Input: part model. Units: mm. Frame: model coordinates. A direction names the side the tool comes from. Give positions to 0.01 mm unless a question says otherwise; leave off trailing zeros. Loops run counter-clockwise (first coordinate to the right, second up) from the corner with the lowest first, then second, coordinate; pieces in that order, holes last. Notation, with made-up numbers: M 1,29 L 15,29 A17 ccw 15,39 Z; hole C -36.5,-12 d11. An arc over 180 degrees is marked long. Use CSV: the item, a comma, the result in double quotes. Start each with the question number.
Q1. Reachability of faces 4 (the flat face through (9.525, 0, 266)), 5 (the flat face through (-10, -2, 539.75)) from +Z, -Z, +X, -X, +Y, -Y: full face, straight path, thin tool, end or side. Return the list, or none.
Q2. Material intervals for line 1 along X through (y, z) = (6, 145) (3 decimals); line 2 along X through (y, z) = (-23, 533); line 3 along Y through (x, z) = (2, 227) (3 decimals), sorted ascending.
Q3. Pin query (flat end, axial travel): pin 1 (2 mm diameter, centred on y = 0, z = 148.968, fed in from -X) (3 decimals). Return the tip coordinate at first contact, or that it passes through.
Q4. Pull-direction query (Y, two-part tool) for faces 1 (the flat face through (-12.7, 0, 266)), 2 (the flat face through (0, 22.225, 266)), 3 (the flat face through (0, 25.4, 266)); classes: released by +Y, released by -Y, zero draft, split by the parting line, or undercut.
Q5. Section A-A, the plane z = 371.5. Output: boundary loops of the cut face in (x, y) (3 decimals).
Q6. Section B-B, the plane y = -11.5. Output: boundary loops of the cut face in (x, z) (3 decimals).
from build123d import *

# Parameters (mm, degrees)
SKETCH1_W                       = 25.4
SKETCH1_H                       = 50.8
SKETCH1_W_2                     = 19.05
SKETCH1_H_2                     = 44.45
EXTRUDE_THIN1_DEPTH             = 539.75
F_10_CLEARANCE_HOLE1_D          = 5.1054
M4X0_7_TAPPED_HOLE1_D           = 3.3
M4X0_7_TAPPED_HOLE1_DEPTH       = 3.175
F_1_8_0_13_DIAMETER_HOLE1_D     = 3.302
F_1_8_0_13_DIAMETER_HOLE1_DEPTH = 3.175


with BuildPart() as part:
    # Sketch1 → Extrude-Thin1 (new body)
    with BuildSketch(Plane.XY):
        Rectangle(SKETCH1_W, SKETCH1_H)
        Rectangle(SKETCH1_W_2, SKETCH1_H_2, mode=Mode.SUBTRACT)
    extrude(amount=EXTRUDE_THIN1_DEPTH)

    # #10 Clearance Hole1 (through all)
    with Locations(Plane(origin=(0, 25.4, 0), x_dir=(1, 0, 0), z_dir=(0, 1, 0))):
        with Locations((0, -533.4), (0, -508), (0, -482.6), (0, -6.35), (0, -31.75), (0, -57.15)):
            Hole(F_10_CLEARANCE_HOLE1_D / 2)

    # M4x0.7 Tapped Hole1
    with Locations(Plane.ZY.offset(12.7)):
        with Locations((148.968, 0), (88.968, 0), (28.968, 0), (208.968, 0), (268.968, 0), (328.968, 0), (388.968, 0), (448.968, 0), (508.968, 0)):
            Hole(M4X0_7_TAPPED_HOLE1_D / 2, depth=M4X0_7_TAPPED_HOLE1_DEPTH)

    # 1/8 (0.13) Diameter Hole1
    with Locations(Plane(origin=(0, -25.4, 0), x_dir=(-1, 0, 0), z_dir=(0, -1, 0))):
        with Locations((3.175, -70.358), (-3.175, -95.758), (3.175, -127.508), (-3.175, -152.908), (3.175, -184.658), (3.175, -241.808), (-3.175, -267.208), (2.890210973, -300.584252198), (-3.175, -324.358), (3.175, -356.108), (-3.175, -381.508), (3.175, -413.258), (-3.175, -438.658), (3.175, -470.408), (-3.175, -210.058)):
            Hole(F_1_8_0_13_DIAMETER_HOLE1_D / 2, depth=F_1_8_0_13_DIAMETER_HOLE1_DEPTH)


solid = part.part
A:
1,face 4,"+Z, -Z"
1,face 5,"+Z, +X, -X, +Y, -Y"
2,line 1,"-12.7 to -9.525, 9.525 to 12.7"
2,line 2,"-12.7 to -2.52, 2.52 to 12.7"
2,line 3,"-25.4 to -22.225, 22.225 to 25.4"
3,pin 1,"x = 9.525"
4,face 1,"zero draft"
4,face 2,"undercut"
4,face 3,"released by +Y"
5,outline,"M -12.7,-25.4 L 12.7,-25.4 L 12.7,25.4 L -12.7,25.4 Z; hole M -9.525,-22.225 L 9.525,-22.225 L 9.525,22.225 L -9.525,22.225 Z"
6,outline,"M -12.7,0 L -9.525,0 L -9.525,539.75 L -12.7,539.75 Z; M 9.525,0 L 12.7,0 L 12.7,539.75 L 9.525,539.75 Z"
